```python
from build123d import *

# Parameters (mm, degrees)
RESSALTO_EXTRUS_O1_DEPTH   = 180
RESSALTO_EXTRUS_O1_2_DEPTH = 180
RESSALTO_EXTRUS_O1_3_DEPTH = 180
RESSALTO_EXTRUS_O1_4_DEPTH = 180
RESSALTO_EXTRUS_O2_DEPTH   = 3


with BuildPart() as part:
    # Esbo_o1 → Ressalto-extrus_o1 (new body)
    with BuildSketch(Plane(origin=(0, 0, 0), x_dir=(1, 0, 0), z_dir=(0, 1, 0))):
        Polygon((-25, 10.355339059), (-10.355339059, 25), (-8.234018716, 22.878679656), (-22.878679656, 8.234018716), align=None)
    extrude(amount=RESSALTO_EXTRUS_O1_DEPTH)



with BuildPart() as body_2:
    # Esbo_o1 → Ressalto-extrus_o1 2 (new body)
    with BuildSketch(Plane(origin=(0, 0, 0), x_dir=(1, 0, 0), z_dir=(0, 1, 0))):
        Polygon((10.355339059, 25), (25, 10.355339059), (22.878679656, 8.234018716), (8.234018716, 22.878679656), align=None)
    extrude(amount=RESSALTO_EXTRUS_O1_2_DEPTH)


with BuildPart() as body_3:
    # Esbo_o1 → Ressalto-extrus_o1 3 (new body)
    with BuildSketch(Plane(origin=(0, 0, 0), x_dir=(1, 0, 0), z_dir=(0, 1, 0))):
        Polygon((25, -10.355339059), (10.355339059, -25), (8.234018716, -22.878679656), (22.878679656, -8.234018716), align=None)
    extrude(amount=RESSALTO_EXTRUS_O1_3_DEPTH)


with BuildPart() as body_4:
    # Esbo_o1 → Ressalto-extrus_o1 4 (new body)
    with BuildSketch(Plane(origin=(0, 0, 0), x_dir=(1, 0, 0), z_dir=(0, 1, 0))):
        Polygon((-10.355339059, -25), (-25, -10.355339059), (-22.878679656, -8.234018716), (-8.234018716, -22.878679656), align=None)
    extrude(amount=RESSALTO_EXTRUS_O1_4_DEPTH)


with BuildPart() as part_1:
    add(part.part)

    add(body_2.part)  # Ressalto-extrus_o2 merges body 2

    add(body_3.part)  # Ressalto-extrus_o2 merges body 3

    add(body_4.part)  # Ressalto-extrus_o2 merges body 4
    # Esbo_o2 → Ressalto-extrus_o2 (add)
    with BuildSketch(Plane(origin=(0, 180, 0), x_dir=(1, 0, 0), z_dir=(0, 1, 0))):
        Polygon((-10.355339059, 25), (10.355339059, 25), (25, 10.355339059), (25, -10.355339059), (10.355339059, -25), (-10.355339059, -25), (-25, -10.355339059), (-25, 10.355339059), align=None)
    extrude(amount=RESSALTO_EXTRUS_O2_DEPTH)


solid = part_1.part
```
The model under review builds one solid part; all positions refer to its coordinate system, in mm. A direction names the side the tool comes from. Round coordinates to 2 decimals unless told otherwise and drop trailing zeros. Order: outer loops, then holes, each group sorted by start corner. A loop starts at its lowest first (then second) coordinate and runs counter-clockwise, first axis right, second up. Notation, with made-up numbers: (57.5, 2.25) -> (77.5, 2.25) arc R16 cw to (77.5, 12.25) -> close; hole circle Ø11 at (-4, 28.25). An arc over 180 degrees is marked (long way). Use a Markdown table: item, result.
Q1. Mouldability with a two-part tool opening along X and no side actions: class faces 1 (the flat face through (15.66, 88.74, -15.45)), 2 (the flat face through (-17, 0, -17)), 3 (the flat face through (-17.575, 90.219, 17.78)), 4 (the flat face through (-15.66, 88.74, 15.45)) as +X half, -X half, draft (parallel to the pull), parting line (faces both ways), or undercut.
Values:
| item | result |
|---|---|
| face 1 | undercut |
| face 2 | draft |
| face 3 | -X half |
| face 4 | undercut |
Q2. Clearance check with flat-ended pins moving along their axes: P1, Ø1, axis at x = 15.5, z = 12.5, coming from the -Y side; P2, Ø4, axis at x = -13, y = 68.5, coming from the -Z side; P3, Ø1, axis at x = -8, y = 37, coming from the +Z side. State where each tip first meets the part, or that it passes through.
Values:
| item | result |
|---|---|
| P1 | stops at y = 180 |
| P2 | stops at z = -24.36 |
| P3 | stops at z = 23.14 |
Q3. For line 1 (Y direction, x = 9.5, z = 17.5); line 2 (X direction, y = 161.5, z = 15.5); line 3 (Z direction, x = 11.5, y = 133), list the stretches that pass through material, from the lowest coordinate up.
Values:
| item | result |
|---|---|
| line 1 | y = 180 to 183 |
| line 2 | x = -19.86 to -15.61, 15.61 to 19.86 |
| line 3 | z = -23.86 to -19.61, 19.61 to 23.86 |
Q4. We need section A-A on y = 141. Write out the cut boundary in (x, z).
Values:
| item | result |
|---|---|
| outline | (-25, -10.36) -> (-10.36, -25) -> (-8.23, -22.88) -> (-22.88, -8.23) -> close; (-25, 10.36) -> (-22.88, 8.23) -> (-8.23, 22.88) -> (-10.36, 25) -> close; (8.23, -22.88) -> (10.36, -25) -> (25, -10.36) -> (22.88, -8.23) -> close; (8.23, 22.88) -> (22.88, 8.23) -> (25, 10.36) -> (10.36, 25) -> close |
Q5. We need section B-B on x = -20. Write out the cut boundary in (y, z).
Values:
| item | result |
|---|---|
| outline | (0, -15.36) -> (183, -15.36) -> (183, 15.36) -> (0, 15.36) -> (0, 11.11) -> (180, 11.11) -> (180, -11.11) -> (0, -11.11) -> close |
Q6. We need section C-C on z = 16.5. Write out the cut boundary in (x, y).
Values:
| item | result |
|---|---|
| outline | (-18.86, 0) -> (-14.61, 0) -> (-14.61, 180) -> (14.61, 180) -> (14.61, 0) -> (18.86, 0) -> (18.86, 183) -> (-18.86, 183) -> close |
Q7. We need section D-D on z = 4. Write out the cut boundary in (x, y), then the cut area to 3 significant figures.
Values:
| item | result |
|---|---|
| outline | (-25, 180) -> (25, 180) -> (25, 183) -> (-25, 183) -> close |
| area | 150 mm^2 |
Q8. Tool access review of faces 5 (the flat face through (17, 0, -17)), 6 (the flat face through (-15.45, 88.74, -15.66)): name each direction out of +Z, -Z, +X, -X, +Y, -Y from which nothing blocks a thin tool from reaching the whole face with its end or side.
Values:
| item | result |
|---|---|
| face 5 | +Z, -Z, +X, -X, -Y |
| face 6 | -Y |
